Part model, mm, in its own coordinate system. Coordinates: 2 decimals unless noted, no trailing zeros. Loops run counter-clockwise (first coordinate to the right, second up) from the corner with the lowest first, then second, coordinate; pieces in that order, holes last. Notation, with made-up numbers: M 3,14 L 42,14 A20 ccw 42,22 Z; hole C -37,-30 d9. An arc over 180 degrees is marked long. Use a Markdown table: item, result. Add a question column.
1) Band-saw the part on C-C (z = 1). State how many separate pieces and enclosed holes the cut face has, plus the area to 3 significant figures.
2) Band-saw the part on D-D (x = -100.5). List the corners of the cut face in (y, z).
3) Wall check: probe 1 along Y at (x, z) = (-73, 2); probe 2 along Y at (x, z) = (-56.5, 1.25); probe 3 along X at (y, z) = (124, 3). Give the ranges that are in metal, low to high. Write a range as from..to.
4) Band-saw the part on A-A (y = 147). List the corners of the cut face in (x, z), plus the area to 3 significant figures.
5) Band-saw the part on B-B (x = -76.2). List the corners of the cut face in (y, z).
6) Pin check, flat tips, straight feed: pin 1 Ø1.6 at (y, z) = (9, 1.5) entering from -X; pin 2 Ø2.5 at (y, z) = (13.5, 2.5) entering from +X; pin 3 Ø2 at (x, z) = (-25, 3) entering from -Y. Stop position of each tip, or through.
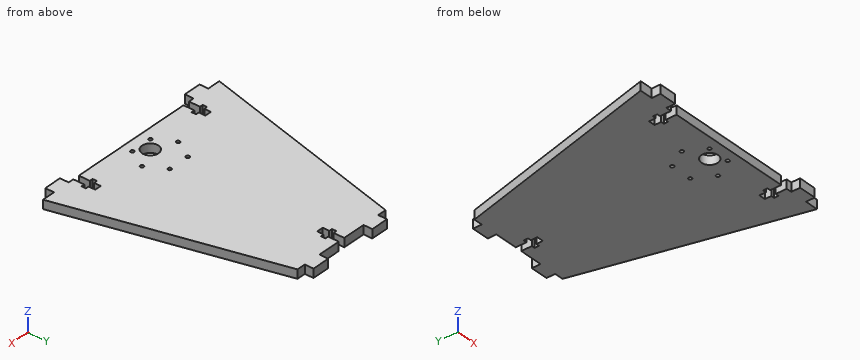
from build123d import *

# Parameters (mm, degrees)
BOSS_EXTRUDE1_DEPTH = 6.35
SKETCH4_R           = 5.969
SKETCH4_R_2         = 1.27
CUT_EXTRUDE3_DEPTH  = 6.35


with BuildPart() as part:
    # Sketch2 → Boss-Extrude1 (new body)
    with BuildSketch(Plane.XY):
        Polygon((0, 0), (-9.525, 0), (-9.525, -6.35), (-22.225, -6.35), (-22.225, 0), (-26.19375, 0), (-26.19375, 7.9375), (-23.8125, 7.9375), (-23.8125, 11.1125), (-26.19375, 11.1125), (-26.19375, 15.875), (-30.95625, 15.875), (-30.95625, 11.1125), (-33.3375, 11.1125), (-33.3375, 7.9375), (-30.95625, 7.9375), (-30.95625, 0), (-121.44375, 0), (-121.44375, 7.9375), (-119.0625, 7.9375), (-119.0625, 11.1125), (-121.44375, 11.1125), (-121.44375, 15.875), (-126.20625, 15.875), (-126.20625, 11.1125), (-128.5875, 11.1125), (-128.5875, 7.9375), (-126.20625, 7.9375), (-126.20625, 0), (-130.175, 0), (-130.175, -6.35), (-142.875, -6.35), (-142.875, 0), (-152.4, 0), (-114.3, 152.4), (-107.95, 152.4), (-107.95, 158.75), (-95.25, 158.75), (-95.25, 152.4), (-78.58125, 152.4), (-78.58125, 144.685169992), (-80.9625, 144.685169992), (-80.9625, 141.510169992), (-78.58125, 141.510169992), (-78.58125, 136.747669992), (-73.81875, 136.747669992), (-73.81875, 141.510169992), (-71.4375, 141.510169992), (-71.4375, 144.685169992), (-73.81875, 144.685169992), (-73.81875, 152.4), (-57.15, 152.4), (-57.15, 158.75), (-44.45, 158.75), (-44.45, 152.4), (-38.1, 152.4), align=None)
    extrude(amount=BOSS_EXTRUDE1_DEPTH)

    # Sketch4 → Cut-Extrude3 (cut)
    with BuildSketch(Plane(origin=(0, 0, 0), x_dir=(-1, 0, 0), z_dir=(0, 0, -1))):
        with Locations((76.2, 13.843)):
            Circle(SKETCH4_R)
        with Locations((68.3895, 34.483182833)):
            Circle(SKETCH4_R_2)
        with Locations((84.0105, 34.483182833)):
            Circle(SKETCH4_R_2)
        with Locations((91.821, 20.955)):
            Circle(SKETCH4_R_2)
        with Locations((84.0105, 7.426817167)):
            Circle(SKETCH4_R_2)
        with Locations((68.3895, 7.426817167)):
            Circle(SKETCH4_R_2)
        with Locations((60.579, 20.955)):
            Circle(SKETCH4_R_2)
    extrude(amount=-CUT_EXTRUDE3_DEPTH, mode=Mode.SUBTRACT)


solid = part.part
Entries:
| question | item | result |
|---|---|---|
| 1 | separate pieces | 1 |
| 1 | enclosed holes | 7 |
| 1 | area | 17,300 mm2 |
| 2 | outline | M 0,0 L 158.75,0 L 158.75,6.35 L 0,6.35 Z |
| 3 | probe 1 | 0..8.8, 18.88..141.51, 144.69..152.4 |
| 3 | probe 2 | 0..158.75 |
| 3 | probe 3 | -121.4..-31 |
| 4 | outline | M -115.65,0 L -78.58,0 L -78.58,6.35 L -115.65,6.35 Z; M -73.82,0 L -36.75,0 L -36.75,6.35 L -73.82,6.35 Z |
| 4 | area | 471 mm2 |
| 5 | outline | M 0,0 L 7.87,0 L 7.87,6.35 L 0,6.35 Z; M 19.81,0 L 136.75,0 L 136.75,6.35 L 19.81,6.35 Z |
| 6 | pin 1 | x = -150.35 |
| 6 | pin 2 | x = -3.06 |
| 6 | pin 3 | y = 0 |
